Source: CAD feature listing. Evaluate the final solid. Frame: model axes, mm. A direction names the side the tool comes from. Give positions to 0.01 mm unless a question says otherwise; leave off trailing zeros. Loops run counter-clockwise (first coordinate to the right, second up) from the corner with the lowest first, then second, coordinate; pieces in that order, holes last. Notation, with made-up numbers: (28, 72) -> (56, 72) arc R22 ccw to (56, 94) -> close; hole circle Ø10 at (21.5, -7.5). An arc over 180 degrees is marked (long way). Put each result on its own line as item: value.
Autodesk Inventor part; units mm, degrees
ref_plane "YZ Plane" through (0, 0, 0) normal (1, 0, 0) x (0, 1, 0)
ref_plane "XZ Plane" through (0, 0, 0) normal (0, 1, 0) x (-1, 0, 0)
ref_plane "XY Plane" through (0, 0, 0) normal (0, 0, 1) x (1, 0, 0)
sketch "Sketch1" plane through (0, 0, 0) normal (0, 1, 0) x (-1, 0, 0)
  line L0 (0, 0) -> (0, -54)
  line L1 (0, -54) -> (5, -54)
  line L2 (5, -54) -> (5, -58)
  line L3 (5, -58) -> (0, -58)
  line L4 (0, -58) -> (0, -54)
  line L5 (0, 0) -> (3, 0)
  line L6 (3, 0) -> (3, 4)
  line L7 (3, 4) -> (0, 4)
  line L8 (0, 4) -> (0, 0)
  line L9 (3, 0) -> (0, 0)
  line L10 (0, 0) -> (0, -54)
  line L11 (0, -54) -> (3, -54)
  line L12 (3, -54) -> (3, 0)
  line L13 (3, 4) -> (43, 4)
  line L14 (43, 4) -> (43, 0)
  line L15 (43, 0) -> (3, 0)
  line L16 (3, 0) -> (3, 4)
  line L17 (3, -54) -> (43, -54)
  line L18 (43, -54) -> (43, -58)
  line L19 (43, -58) -> (3, -58)
  line L20 (3, -58) -> (3, -54)
  line L21 (0, -27) -> (-82.8143, -27)
  line L22 (-82.8143, -27) -> (-97.578, -27)
  line L23 (0, 4) -> (90, 4) construction
  line L24 (0, 0) -> (80, 0) construction
  line L25 (-84.5723, -27) -> (-84.5723, -17)
  line L26 (-84.5723, -27) -> (-84.5723, -37)
  line L27 (-84.5723, -37) -> (-80.5723, -37)
  line L28 (-80.5723, -37) -> (-80.5723, -17)
  line L29 (-80.5723, -17) -> (-84.5723, -17)
  line L30 (0, 0) -> (-80.5723, -17)
  line L31 (0, -54) -> (-80.5723, -37)
  line L32 (-80.5723, -37) -> (-80.5723, -41)
  line L33 (-80.5723, -41) -> (0, -58)
  line L34 (-84.5723, -37) -> (-80.5723, -41)
  line L35 (-80.5723, -17) -> (-80.5723, -13)
  line L36 (-80.5723, -13) -> (0, 4)
  line L37 (-84.5723, -17) -> (-80.5723, -13)
  line L38 (3, -27) -> (13, -27)
  circle A0 centre (13, -27) radius 28.7924
  line L39 (41.7924, -27) -> (44.7924, -27)
  circle A1 centre (13, -27) radius 31.7924
  point P0 (-85.1718, -27)
  point P1 (-74.1819, -27)
  point P2 (3, 0)
  point P3 (-5.5314, -1.1671)
  point P4 (-5.5314, -52.8329)
  dimension "d0" = 54
  dimension "d1" = 5
  dimension "d2" = 4
  dimension "d3" = 3
  dimension "d4" = 4
  dimension "d5" = 40
  dimension "d6" = 40
  dimension "d32" = 10
  dimension "d34" = 10
  dimension "d35" = 4
  dimension "d36" = 4
  dimension "d37" = 4
  dimension "d41" = 10
  dimension "d42" = 3
  dimension "d58" = 4
extrude "Extrusion1" add sketch "Sketch1" along normal blind 20 contours L5 A0 L0 | L8 A1 L6 L5 | L30 A1 L8 | L0 A0 L21 A1 L30 | A0 L15 | L6 A1 L13 L15 A0 | A1 L30 L35 L36 L8 | L8 L7 L6 A1 | A0 L0 L31 A1 L21 | L6 L13 A1 | L28 L21 L22 L25 L29 | L29 L37 L35 | A0 L1 L0 | L20 A1 L4 L1 | A0 L2 A1 L20 | L1 L2 A0 | A1 L13 L14 L15 | L28 L27 L26 L22 L21 | A1 L4 L33 L32 L31 | L31 L4 A1 | L17 A0 L2 | A1 L2 L3 L20 | L20 L3 L4 A1 | A0 L17 A1 L19 L2 | L32 L34 L27 | A1 L19 L2 | L17 L18 L19 A1
sketch "Sketch2" plane through (-43, 0, 4) normal (0, 0, 1) x (1, 0, 0)
  line L0 (43, 20) -> (0, 20)
  line L1 (0, 20) -> (10, 20)
  line L2 (10, 20) -> (10, 10)
  line L3 (10, 10) -> (0, 10)
  line L4 (0, 10) -> (0, 20)
  circle A0 centre (10, 10) radius 3
  circle A1 centre (10, 10) radius 10
  line L5 (128.1718, 0) -> (128.1718, 20)
  line L6 (128.1718, 10) -> (128.1718, 17)
  line L7 (128.1718, 17) -> (128.1718, 3)
  line L8 (43, 0) -> (0, 0)
  line L9 (128.1718, 3) -> (43, 0)
  line L10 (43, 0) -> (128.1718, 0)
  line L11 (128.1718, 0) -> (128.1718, 3)
  line L12 (43, 20) -> (73.6773, 20)
  line L13 (128.1718, 17) -> (43, 20)
  line L14 (128.1718, 20) -> (43, 20)
  line L15 (43, 20) -> (128.1718, 20)
  line L16 (128.1718, 20) -> (128.1718, 17)
  line L17 (10, 10) -> (0, 10)
  line L18 (0, 10) -> (0, 0)
  line L19 (0, 0) -> (10, 0)
  line L20 (10, 0) -> (10, 10)
  circle A2 centre (10, 10) radius 8
  circle A3 centre (10, 10) radius 6.5
  line L21 (10, 18) -> (10, 16.5)
  circle A4 centre (10, 17.25) radius 1.1
  line L22 (2, 10) -> (3.5, 10)
  circle A5 centre (2.75, 10) radius 1.1
  line L23 (10, 3.5) -> (10, 2)
  circle A6 centre (10, 2.75) radius 1.1
  line L24 (16.5, 10) -> (18, 10)
  circle A7 centre (17.25, 10) radius 1.1
  dimension "d15" = 10
  dimension "d16" = 10
  dimension "d17" = 6
  dimension "d18" = 7
  dimension "d19" = 14
  dimension "d22" = 16
  dimension "d23" = 13
  dimension "d24" = 2.2
  dimension "d25" = 2.2
  dimension "d26" = 2.2
  dimension "d27" = 2.2
extrude "Extrusion2" cut sketch "Sketch2" against normal blind 100 contours L12 L14 L5 L13 | A1 L4 L0 | A4 A2 L2 | L2 A2 A4 | A1 L8 L18 | A2 A4 A3 L2 | L2 A3 A4 A2 | A5 A2 L3 | L3 A2 A5 | L5 L10 L9 | A3 A4 L2 | L2 A4 A3 | A7 A2 | A2 L24 A3 A7 | A5 A3 L3 A2 | A6 A2 L20 | L20 A2 A6 | L3 A3 A5 A2 | A2 A7 A3 L24 | A3 A7 | A5 L3 A3 | A2 A6 A3 L20 | L20 A3 A6 A2 | L3 A5 A3 | A0 L20 L2 | L2 L3 A0 | A3 A6 L20 | L20 A6 A3 | L20 A0 L3
sketch "Sketch3" plane through (80.5723, 2.838, -17) normal (-1, 0, 0) x (0, 0, 1)
  line L0 (0, 14.324) -> (-20, 14.324)
  line L1 (-20, 14.1831) -> (0, 14.1831)
  line L2 (0, 14.324) -> (-20, 14.1831)
  line L3 (-10, 14.2536) -> (-10, 0)
  line L4 (-20, 0) -> (0, 0)
  line L5 (-14, 0.6268) -> (-6, 0.6268)
  line L6 (-6, 0.6268) -> (-6, 13.6268)
  line L7 (-6, 13.6268) -> (-14, 13.6268)
  line L8 (-14, 13.6268) -> (-14, 0.6268)
  line L9 (-14, 0.6268) -> (-6, 13.6268) construction
  line L10 (-6, 0.6268) -> (-14, 13.6268) construction
  line L11 (-14, 0.6268) -> (-10, 0.6268)
  line L12 (-10, 0.6268) -> (-10, 2.4268)
  line L13 (-10, 2.4268) -> (-14, 2.4268)
  line L14 (-14, 2.4268) -> (-14, 0.6268)
  circle A0 centre (-10, 2.4268) radius 1
  line L15 (-14, 13.6268) -> (-6, 13.6268)
  line L16 (-6, 13.6268) -> (-6, 12.6268)
  line L17 (-6, 12.6268) -> (-14, 12.6268)
  line L18 (-14, 12.6268) -> (-14, 13.6268)
  line L19 (-14, 13.6268) -> (-13, 13.6268)
  line L20 (-13, 13.6268) -> (-13, 0.6268)
  line L21 (-13, 0.6268) -> (-14, 0.6268)
  line L22 (-14, 0.6268) -> (-14, 13.6268)
  line L23 (-6, 13.6268) -> (-7, 13.6268)
  line L24 (-7, 13.6268) -> (-7, 0.6268)
  line L25 (-7, 0.6268) -> (-6, 0.6268)
  line L26 (-6, 0.6268) -> (-6, 13.6268)
  line L27 (-6, 0.6268) -> (-14, 0.6268)
  line L28 (-14, 0.6268) -> (-14, 3.6268)
  line L29 (-14, 3.6268) -> (-6, 3.6268)
  line L30 (-6, 3.6268) -> (-6, 0.6268)
  line L31 (-9.0365, 2.6944) -> (-11, 2.6944)
  line L32 (-11, 2.6944) -> (-11, 4.6268)
  line L33 (-11, 4.6268) -> (-9.0365, 4.6268)
  line L34 (-9.0365, 4.6268) -> (-9.0365, 2.6944)
  line L35 (-6, 13.6268) -> (-7, 13.6268)
  line L36 (-7, 13.6268) -> (-7, 3.6268)
  line L37 (-7, 3.6268) -> (-6, 3.6268)
  line L38 (-6, 3.6268) -> (-6, 13.6268)
  point P0 (17, -2.838)
  point P1 (-10, 7.1268)
  point P2 (-9.0365, 3.6268)
  point P3 (-7, 12.6268)
  point P4 (-13, 12.6268)
  point P5 (-13, 3.6268)
  point P6 (-11, 3.6268)
  dimension "d46" = 2
  dimension "d38" = 8
  dimension "d39" = 13
  dimension "d44" = 4
  dimension "d45" = 1.8
  dimension "d47" = 1
  dimension "d48" = 1
  dimension "d49" = 1
  dimension "d50" = 3
  dimension "d51" = 4
fillet "Fillet1" radius 4 4 edges at (80.5723, 10, -41) (80.5723, 10, -13) (80.5723, 10, -37) (80.5723, 10, -17)
fillet "Fillet2" radius 4 2 edges at (5.5314, 10, -52.8329) (5.5314, 10, -1.1671)
extrude "Extrusion3" cut sketch "Sketch3" against normal blind 20 contours L17 L24 L29 L34 L33 L3 | L3 L33 L32 L29 L20 L17 | A0 L31 L3 | L3 L31 A0 | L31 A0 L3 | L3 L13 A0 L31 | L13 L3 A0
extrude "Extrusion4" cut sketch "Sketch3" against normal blind 2 contours L7 L24 L17 L3 | L3 L17 L20 L7 | L7 L6 L17 L24 | L20 L17 L8 L7 | L33 L34 L29 L3 | L3 L29 L32 L33 | L17 L6 L29 L24 | L20 L29 L8 L17 | L29 L34 A0 L3 | L3 A0 L31 L32 L29 | L29 L6 L5 L24 | L24 L5 L3 A0 L34 L29 | L29 L32 L31 A0 L13 L20 | L20 L13 L8 L29 | A0 L31 L3 | L3 L31 A0 | L20 L5 L8 L13 | L13 A0 L3 L5 L20 | L31 A0 L3 | L3 L13 A0 L31 | L13 L3 A0
sketch "Sketch4" plane through (84.5723, 17.0211, -17) normal (0.0352, 0.9994, 0) x (0.9994, -0.0352, 0)
  ellipse E0 centre (-97.6328, 10) end of major axis (-129.4449, 10) minor radius 31.7924 (-70.8385, -7.1379) -> (-70.8385, 27.1379) ccw
  line L0 (-97.6328, 10) -> (-62.4593, 10)
  line L1 (-62.4593, 10) -> (-62.4593, 13)
  line L2 (-62.4593, 13) -> (-97.6328, 13)
  line L3 (-97.6328, 13) -> (-97.6328, 10)
  line L4 (-97.6328, 10) -> (-62.4593, 10)
  line L5 (-62.4593, 10) -> (-62.4593, 7)
  line L6 (-62.4593, 7) -> (-97.6328, 7)
  line L7 (-97.6328, 7) -> (-97.6328, 10)
  point P0 (-83.9208, -17)
  point P1 (-62.4593, 10)
  dimension "d59" = 3
  dimension "d60" = 3
extrude "Extrusion6" cut sketch "Sketch4" against normal blind 3
fillet "Fillet3" radius 1 2 edges at (17.1431, 19.3962, -30) (17.1431, 19.3962, -24)
properties part number "calf_2"
(1) Line query: probe 1 along Y at (x, z) = (83.75, -27); probe 2 along Y at (x, z) = (-33, 2.8); probe 3 along Z at (x, y) = (-8.5, 2.25). Output: solid intervals per line, ascending. Write a range as from..to.
Calculated:
probe 1: y = 2.95..4.26, 6.26..7.46, 15.46..17.05
probe 2: y = 0..1.65, 3.85..7, 13..16.15, 18.35..20
probe 3: z = -58..-54, 0..4
(2) Reachability of faces 5 (the flat face through (47.269, 9.869, -44.027)), 6 (the flat face through (-23, 10, 0)), 7 (the flat face through (82.572, 7, -27)), 8 (the flat face through (-16, 20, 2)), 9 (the cylindrical face through (-31.95, 3.08, -55.97)) from +Z, -Z, +X, -X, +Y, -Y: full face, straight path, thin tool, end or side. Return the list, or none.
Calculated:
face 5: +Y, -Y
face 6: -X, +Y, -Y
face 7: none
face 8: +Z, -Z, +X, -X, +Y
face 9: +Z, -Z
(3) Section A-A on x = -16. Return loops of the section in (y, z), then the cut area to 3 significant figures.
Calculated:
outline: (0, -58) -> (20, -58) -> (20, -54) -> (0, -54) -> close; (0, 0) -> (20, 0) -> (20, 4) -> (0, 4) -> close
area: 160 mm²
(4) Section B-B on x = 49.5. Return loops of the section in (y, z), then the cut area to 3 significant figures.
Calculated:
outline: (1.74, -47.56) -> (18.26, -47.56) -> (18.26, -43.56) -> (1.74, -43.56) -> close; (1.74, -10.44) -> (18.26, -10.44) -> (18.26, -6.44) -> (1.74, -6.44) -> close
area: 132 mm²
(5) Draft query along Z for faces 1 (the cylindrical face through (-39.234, 9.579, 2.028)), 2 (the flat face through (-21, 10, 4)), 3 (the flat face through (-23, 10, -54)), 4 (the flat face through (47.269, 9.869, -9.973)). Return one class per face: released by +Z, released by -Z, zero draft, split by the parting line, or undercut.
Calculated:
face 1: zero draft
face 2: released by +Z
face 3: undercut
face 4: undercut
(6) First-contact query: P1, Ø8, axis at x = 21, y = 7, coming from the +Z side; P2, Ø6, axis at x = 15, z = -28.5, coming from the +Y side; P3, Ø1.6, axis at x = 82, y = 12, coming from the +Z side. Flat tips, straight axial feed; report the tip coordinate or a pass-through.
Calculated:
P1: stops at z = 0.41
P2: stops at y = 19.46
P3: stops at z = -13.64
